Input: part model. Units: mm. Frame: model coordinates. A direction names the side the tool comes from. Round coordinates to 2 decimals unless told otherwise and drop trailing zeros. Loops run counter-clockwise (first coordinate to the right, second up) from the corner with the lowest first, then second, coordinate; pieces in that order, holes last. Notation, with made-up numbers: (42.25, 70) -> (73.25, 70) arc R18 ccw to (73.25, 91) -> close; hole circle Ø1 at (-38.5, 51). An arc over 180 degrees is marked (long way). Answer as a JSON object with one key per item and string values. Group by question number.
Item 1: Section query B-B on x = -40. Return loops of the section in (y, z).
Item 2: Pin query (flat end, axial travel): pin 1 (10 mm diameter, centred on x = -26.5, y = 54.5, fed in from +Z); pin 2 (12 mm diameter, centred on x = -43.5, y = 11, fed in from +Z); pin 3 (5 mm diameter, centred on x = -45, z = -45, fed in from +Y). Return the tip coordinate at first contact, or that it passes through.
Item 3: Set-up query: faces 4 (the flat face through (-50, 17, -25)), 5 (the cylindrical face through (-5.466, 4.056, -46.478)), 6 (the flat face through (-47, 35, -25)). Return all of +Z, -Z, +X, -X, +Y, -Y with unobstructed straight access to the full face (end or side cutting, diameter ignored); none if empty.
Item 4: Draft query along X for faces 1 (the cylindrical face through (-12.62, 49.3, -5.89)), 2 (the cylindrical face through (-43.487, 4.056, -4.664)), 3 (the flat face through (0, 17, -25)). Return one class per face: released by +X, released by -X, zero draft, split by the parting line, or undercut.
Item 5: Section query C-C on y = 50.5. Return loops of the section in (x, z).
Item 6: Material intervals for line 1 (Z direction, x = -45, y = 2.5); line 2 (Z direction, x = -5, y = 8.5), sorted ascending. Write a range as [from, to].
Item 7: Section query A-A on z = -18. Return loops of the section in (x, y).
Autodesk Inventor part; units mm, degrees
ref_plane "YZ Plane" through (0, 0, 0) normal (1, 0, 0) x (0, 1, 0)
ref_plane "XZ Plane" through (0, 0, 0) normal (0, 1, 0) x (-1, 0, 0)
ref_plane "XY Plane" through (0, 0, 0) normal (0, 0, 1) x (1, 0, 0)
sketch "スケッチ1" plane through (0, 0, 0) normal (0, 1, 0) x (-1, 0, 0)
  line L0 (0, 0) -> (50, 0)
  line L1 (50, 0) -> (50, -50)
  line L2 (50, -50) -> (0, -50)
  line L3 (0, -50) -> (0, 0)
  dimension "d0" = 50
  dimension "d1" = 50
extrude "押し出し1" add sketch "スケッチ1" along normal blind 35
sketch "スケッチ2" plane through (0, 35, 0) normal (0, 1, 0) x (1, 0, 0)
  circle A0 centre (-24.4444, 24.4444) radius 22
  point P0 (0, 0)
  dimension "d4" = 44
extrude "押し出し2" add sketch "スケッチ2" along normal blind 29
fillet "フィレット1" radius 5 4 edges at (-50, 17.5, 0) (0, 17.5, 0) (0, 17.5, -50) (-50, 17.5, -50)
sketch "スケッチ3" plane through (0, 0, 0) normal (0, -1, 0) x (1, 0, 0)
  arc A0 (-50, -45) -> (-45, -50) centre (-45, -45) ccw
  line L0 (-5, -50) -> (-45, -50)
  arc A1 (-5, -50) -> (0, -45) centre (-5, -45) ccw
  line L1 (0, -5) -> (0, -45)
  arc A2 (0, -5) -> (-5, 0) centre (-5, -5) ccw
  line L2 (-45, 0) -> (-5, 0)
  arc A3 (-45, 0) -> (-50, -5) centre (-45, -5) ccw
  line L3 (-50, -45) -> (-50, -5)
  point P0 (0, 0)
hole "穴1" at (-5, 0, -5) at (-5, 0, -45) at (-45, 0, -45) at (-45, 0, -5) direction (0, 1, 0) diameter 3.1 depth 8 tip angle 118
properties part number "LiDAR_un" material "ABS プラスチック"
Solved:
{
 "1": {"outline": "(0, -50) -> (35, -50) -> (35, -40) -> (64, -40) -> (64, -8.89) -> (35, -8.89) -> (35, 0) -> (0, 0) -> close"},
 "2": {"pin 1": "z = -2.44", "pin 2": "z = 0", "pin 3": "y = 35"},
 "3": {"face 4": "+Z, -Z, -X, +Y, -Y", "face 5": "-Y", "face 6": "+Y"},
 "4": {"face 1": "split by the parting line", "face 2": "undercut", "face 3": "released by +X"},
 "5": {"outline": "circle Ø44 at (-24.44, -24.44)"},
 "6": {"line 1": "[-50, -46.55], [-43.45, -6.55], [-3.45, 0]", "line 2": "[-50, -45.72], [-44.28, -5.72], [-4.28, 0]"},
 "7": {"outline": "(-50, 0) -> (0, 0) -> (0, 35) -> (-3.41, 35) -> (-3.41, 64) -> (-45.48, 64) -> (-45.48, 35) -> (-50, 35) -> close"}
}
